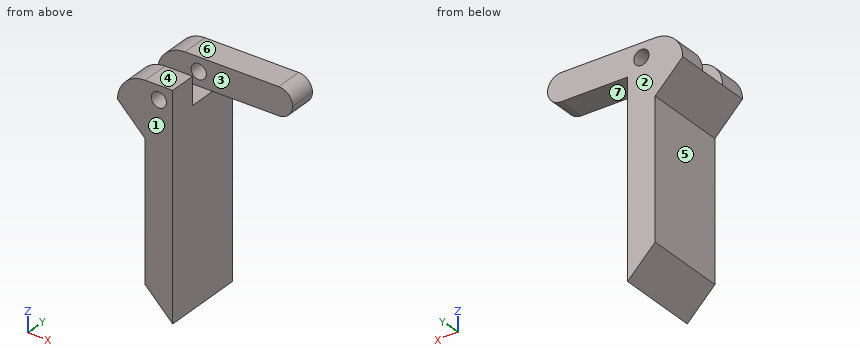
```python
from build123d import *

# Parameters (mm, degrees)
F0_W      = 10
F0_H      = 15
F1_DEPTH  = 5
F2_DEPTH  = 5
F3_R      = 1.375
F4_DEPTH  = 15.001
F5_W      = 5
F5_H      = 5
F6_DEPTH  = 10.001
F7_W      = 5
F7_H      = 5
F8_DEPTH  = 14.5
F9_W      = 5
F9_H      = 15
F10_DEPTH = 30
F11_R     = 2.49999
F12_SIZE  = 4.99999
F13_R     = 5
F14_SIZE  = 4.99999


# Not quite as in the source:
# - a fillet or chamfer is up to 0.001 mm smaller than in the source, because OpenCascade refuses the exact size


with BuildPart() as f1:
    # F0 (on Top) → F1 (new body)
    with BuildSketch(Plane.XY):
        with Locations((-26.6721312702, -21.5040988475)):
            Rectangle(F0_W, F0_H)
    extrude(amount=F1_DEPTH)

    # F2 (add): a face of the model
    f2_faces = [f1.faces().sort_by_distance(p)[0] for p in [
        (-26.6721312702, -21.5040988475, 5),
    ]]
    extrude(f2_faces, amount=F2_DEPTH)

    # F3 (on face) → F4 (cut, through all)
    with BuildSketch(Plane.XZ.offset(29.0040988475)):
        with Locations((-24.1721312702, 7.5)):
            Circle(F3_R)
    extrude(amount=-F4_DEPTH, mode=Mode.SUBTRACT)

    # F5 (on face) → F6 (cut, through all)
    with BuildSketch(Plane.YZ.offset(-21.6721312702)):
        with Locations((-21.5040988475, 7.5)):
            Rectangle(F5_W, F5_H)
    extrude(amount=-F6_DEPTH, mode=Mode.SUBTRACT)

    # F7 (on face) → F8 (join)
    with BuildSketch(Plane.YZ.offset(-21.6721312702)):
        with Locations((-16.5040988475, 7.5)):
            Rectangle(F7_W, F7_H)
    extrude(amount=F8_DEPTH)

    # F9 (on face) → F10 (join)
    with BuildSketch(Plane(origin=(0, 0, 0), x_dir=(1, 0, 0), z_dir=(0, 0, -1))):
        with Locations((-24.1721312702, 21.5040988475)):
            Rectangle(F9_W, F9_H)
    extrude(amount=F10_DEPTH)

    # F11 (radius 2.5 in the source; OpenCascade refuses exactly that, so slightly less here)
    f11_edges = [f1.edges().sort_by_distance(p)[0] for p in [
        (-7.172131, -16.504099, 10),
        (-7.172131, -16.504099, 5),
    ]]
    fillet(f11_edges, radius=F11_R)

    # F12 (size 5 in the source; OpenCascade refuses exactly that, so slightly less here)
    f12_edges = [f1.edges().sort_by_distance(p)[0] for p in [
        (-31.672131, -21.504099, 0),
    ]]
    chamfer(f12_edges, length=F12_SIZE)

    # F13
    f13_edges = [f1.edges().sort_by_distance(p)[0] for p in [
        (-31.672131, -16.504099, 10),
        (-31.672131, -26.504099, 10),
    ]]
    fillet(f13_edges, radius=F13_R)

    # F14 (size 5 in the source; OpenCascade refuses exactly that, so slightly less here)
    f14_edges = [f1.edges().sort_by_distance(p)[0] for p in [
        (-26.672131, -21.504099, -30),
    ]]
    chamfer(f14_edges, length=F14_SIZE)


solid = f1.part
```
Verification items for the finished model (mm, model axes). Face numbers are marked on the shaded views. A direction names the side the tool comes from. Coordinates: 2 decimals unless noted, no trailing zeros. Loops run counter-clockwise (first coordinate to the right, second up) from the corner with the lowest first, then second, coordinate; pieces in that order, holes last. Notation, with made-up numbers: (14.5, 44.25) - (20.5, 44.25) arc R29 cw to (20.5, 76.25) - close; hole circle Ø9 at (22, -38.5). An arc over 180 degrees is marked (long way). Put each result on its own line as item: value.
Item 1: Set-up check for the marked faces 5, 6 and 7: record each of +Z, -Z, +X, -X, +Y, -Y from which the full face is reachable in a straight line by a thin tool's end or side.
Conclusion:
face 5: -Z, -X, +Y, -Y
face 6: +Z, +X, -X, +Y, -Y
face 7: -Z, +X, +Y, -Y
Item 2: Draft check along Y on the marked faces 1, 2, 3 and 4. Enter one of: pulls with the +Y half, pulls with the -Y half, needs draft (parallel to the pull), parting line crosses it, or undercut.
Conclusion:
face 1: pulls with the -Y half
face 2: pulls with the +Y half
face 3: undercut
face 4: needs draft
Item 3: Section check C-C (z = 7). Enter the section's corners in (x, y).
Conclusion:
outline: (-31.25, -29) - (-25.45, -29) - (-25.45, -24) - (-31.25, -24) - close; (-31.25, -19) - (-25.45, -19) - (-25.45, -14) - (-31.25, -14) - close; (-22.89, -29) - (-21.67, -29) - (-21.67, -24) - (-22.89, -24) - close; (-22.89, -19) - (-7.22, -19) - (-7.22, -14) - (-22.89, -14) - close
Item 4: Section check B-B (x = -23.5). Enter the section's corners in (y, z).
Conclusion:
outline: (-29, -28.17) - (-14, -28.17) - (-14, 6.3) - (-19, 6.3) - (-19, 5) - (-24, 5) - (-24, 6.3) - (-29, 6.3) - close; (-29, 8.7) - (-24, 8.7) - (-24, 10) - (-29, 10) - close; (-19, 8.7) - (-14, 8.7) - (-14, 10) - (-19, 10) - close
Item 5: Gauge pin test, flat ends, axial feed: pin 1 Ø3 at (y, z) = (-26, -5.5) entering from -X; pin 2 Ø1.5 at (y, z) = (-23, 1.5) entering from +X; pin 3 Ø1.5 at (x, y) = (-15.5, -15.5) entering from -Z. Record the tip position at first contact, or that the pin passes through.
Conclusion:
pin 1: stops at x = -26.67
pin 2: stops at x = -21.67
pin 3: stops at z = 5
Item 6: Scan lines: line 1 along Y through (x, z) = (-26.25, 7); line 2 along Z through (x, y) = (-17.75, -15.5); line 3 along X through (y, z) = (-17.5, -16.5). Record each from-to range of solid material in increasing order.
Conclusion:
line 1: y = -29 to -24, -19 to -14
line 2: z = 5 to 10
line 3: x = -26.67 to -21.67
